Read the model definition and answer for the solid it produces. Units are mm, in the model's axes. Give positions to 0.01 mm unless a question says otherwise; leave off trailing zeros. Write each loop counter-clockwise with the first axis right and the second up, starting at its lowest first coordinate (ties: lowest second). Pieces come first, ordered by that corner, then holes. Notation, with made-up numbers: M 49.25,37.5 L 71.25,37.5 A30 ccw 71.25,66.5 Z; hole C 82.25,-6 d9. An arc over 180 degrees is marked long. Put each result on its own line as item: value.
from build123d import *

# Parameters (mm, degrees)
SKETCH_1_W          = 164
SKETCH_1_H          = 22.5
EXTRUDE_1_DEPTH     = 24
CUT_EXTRUDE_1_DEPTH = 24
SKETCH_3_W          = 55
SKETCH_3_H          = 10
CUT_EXTRUDE_2_DEPTH = 3


with BuildPart() as part:
    # 草图1 → 凸台-拉伸1 (new body)
    with BuildSketch(Plane.XY):
        with Locations((82, 11.25)):
            Rectangle(SKETCH_1_W, SKETCH_1_H)
    extrude(amount=EXTRUDE_1_DEPTH)

    # 草图2 → 切除-拉伸1 (cut)
    with BuildSketch(Plane.XY.offset(24)):
        with BuildLine():
            ThreePointArc((0, 11.25), (3.295048712, 19.204951288), (11.25, 22.5))
            Line((11.25, 22.5), (0, 22.5))
            Line((0, 22.5), (0, 11.25))
        make_face()
        with BuildLine():
            ThreePointArc((11.25, 0), (3.295048712, 3.295048712), (0, 11.25))
            Line((0, 11.25), (0, 0))
            Line((0, 0), (11.25, 0))
        make_face()
        with BuildLine():
            Line((164, 22.5), (152.75, 22.5))
            ThreePointArc((152.75, 22.5), (160.704951288, 19.204951288), (164, 11.25))
            Line((164, 11.25), (164, 22.5))
        make_face()
        with BuildLine():
            Line((164, 0), (164, 11.25))
            ThreePointArc((164, 11.25), (160.704951288, 3.295048712), (152.75, 0))
            Line((152.75, 0), (164, 0))
        make_face()
    extrude(amount=-CUT_EXTRUDE_1_DEPTH, mode=Mode.SUBTRACT)

    # 草图3 → 切除-拉伸2 (cut)
    with BuildSketch(Plane.XY.offset(24)):
        with Locations((82, 11.5)):
            Rectangle(SKETCH_3_W, SKETCH_3_H)
    extrude(amount=-CUT_EXTRUDE_2_DEPTH, mode=Mode.SUBTRACT)


solid = part.part
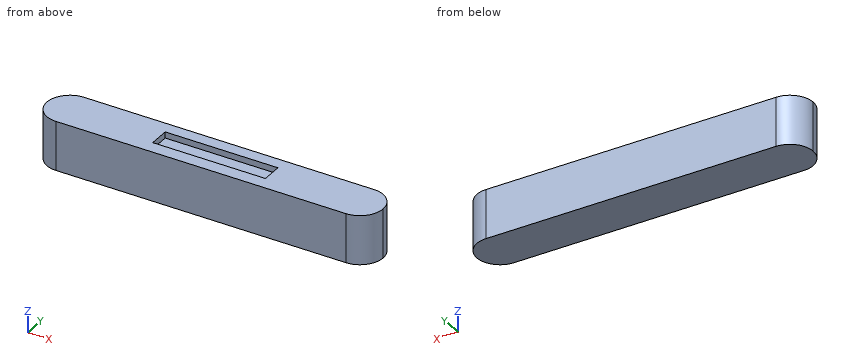
(1) Section B-B on z = 14 is taken. Determine the outline of the cut face in (x, y), and give its area (3 significant figures).
Result:
outline: M 11.25,0 L 152.75,0 A11.25 ccw 152.75,22.5 L 11.25,22.5 A11.25 ccw Z
area: 3,580 mm²
(2) Section D-D on y = 3 is taken. Determine the outline of the cut face in (x, z).
Result:
outline: M 3.6,0 L 160.4,0 L 160.4,24 L 3.6,24 Z
(3) Section A-A on x = 57 is taken. Determine the outline of the cut face in (y, z).
Result:
outline: M 0,0 L 22.5,0 L 22.5,24 L 16.5,24 L 16.5,21 L 6.5,21 L 6.5,24 L 0,24 Z
(4) Straight lines are drawn through the part: line 1 along X through (y, z) = (11, 8.75); line 2 along Z through (x, y) = (61, 7.25); line 3 along X through (y, z) = (2.75, 18.25). For each, find the intervals that lie inside material, in ascending order. Write a range as from..to.
Result:
line 1: x = 0..164
line 2: z = 0..21
line 3: x = 3.88..160.12
(5) Given pin 1 Ø0.9 at (y, z) = (10.5, 22) entering from +X, flat-ended and moving along its own axis, determine where the tip first touches the part or whether it passes through.
Result:
pin 1: stops at x = 164
(6) Section C-C on y = 13 is taken. Determine the outline of the cut face in (x, z), and give its area (3 significant figures).
Result:
outline: M 0.14,0 L 163.86,0 L 163.86,24 L 109.5,24 L 109.5,21 L 54.5,21 L 54.5,24 L 0.14,24 Z
area: 3,760 mm²
